CAD build for the part. Positions are in the model's coordinates, mm. Round coordinates to 2 decimals unless told otherwise and drop trailing zeros. Order: outer loops, then holes, each group sorted by start corner. A loop starts at its lowest first (then second) coordinate and runs counter-clockwise, first axis right, second up. Notation, with made-up numbers: M 50.25,72 L 101.25,72 A22 ccw 101.25,94 Z; hole C 30,-28 d5. An arc over 180 degrees is marked long. Answer as a JSON object with one key per item and string values.
```python
from build123d import *

# Parameters (mm, degrees)
SKETCH1_R               = 0.9271
BOSS_EXTRUDE1_DEPTH     = 1.424
BOSS_EXTRUDE2_OUTLINE_R = 0.9271
BOSS_EXTRUDE2_DEPTH     = 0.6096
CUT_EXTRUDE2_START      = -1.424
SKETCH3_R               = 2
CUT_EXTRUDE2_DEPTH      = 2.848


# Read off the part's stored shape, not the designer's step: Boss-Extrude2
with BuildPart() as part:
    # Sketch1 → Boss-Extrude1 (new, symmetric)
    with BuildSketch(Plane(origin=(0, 0, 0), x_dir=(0, 0, -1), z_dir=(1, 0, 0))):
        with BuildLine():
            Line((-3, 2), (3, 2))
            ThreePointArc((3, 2), (5, 0), (3, -2))
            Line((3, -2), (-3, -2))
            ThreePointArc((-3, -2), (-5, 0), (-3, 2))
        make_face()
        with Locations(Location((-3, 0, 0), (0, 0, 180))):
            Circle(SKETCH1_R, mode=Mode.SUBTRACT)
        with Locations(Location((3, 0, 0), (0, 0, 180))):
            Circle(SKETCH1_R, mode=Mode.SUBTRACT)
    extrude(amount=BOSS_EXTRUDE1_DEPTH, both=True)

    # Boss-Extrude2 outline → Boss-Extrude2 (add)
    with BuildSketch(Plane(origin=(1.424, 0, 0), x_dir=(0, 0, -1), z_dir=(1, 0, 0))):
        with BuildLine():
            Line((-3, -2.5019), (3, -2.5019))
            ThreePointArc((3, -2.5019), (5.5019, 0), (3, 2.5019))
            Line((3, 2.5019), (-3, 2.5019))
            ThreePointArc((-3, 2.5019), (-5.5019, 0), (-3, -2.5019))
        make_face()
        with Locations((-3, 0)):
            Circle(BOSS_EXTRUDE2_OUTLINE_R, mode=Mode.SUBTRACT)
        with Locations((3, 0)):
            Circle(BOSS_EXTRUDE2_OUTLINE_R, mode=Mode.SUBTRACT)
    boss_extrude2 = extrude(amount=BOSS_EXTRUDE2_DEPTH)

    # Mirror1: Boss-Extrude2 across plane
    add(boss_extrude2.mirror(Plane(origin=(0, 0, 0), x_dir=(0, 0, 1), z_dir=(1, 0, 0))))

    # Sketch3 → Cut-Extrude2 (cut)
    with BuildSketch(Plane(origin=(0, 0, 0), x_dir=(0, 0, -1), z_dir=(1, 0, 0)).offset(CUT_EXTRUDE2_START)):
        with BuildLine():
            Line((-3, 2.5019), (3, 2.5019))
            ThreePointArc((3, 2.5019), (5.5019, 0), (3, -2.5019))
            Line((3, -2.5019), (-3, -2.5019))
            ThreePointArc((-3, -2.5019), (-5.5019, 0), (-3, 2.5019))
        make_face()
        with Locations(Location((-3, 0, 0), (0, 0, 180))):
            Circle(SKETCH3_R, mode=Mode.SUBTRACT)
        with Locations(Location((3, 0, 0), (0, 0, 180))):
            Circle(SKETCH3_R, mode=Mode.SUBTRACT)
    extrude(amount=CUT_EXTRUDE2_DEPTH, mode=Mode.SUBTRACT)


solid = part.part
```
Item 1: Two-plate mould, pull along Z, no slides. Class faces 1 (the cylindrical face through (-1.7, -0.1, -5.5)), 2 (the flat face through (-1.424, 0, 0)), 3 (the flat face through (-2.034, 0, 0)): released by +Z, released by -Z, zero draft, split by the parting line, or undercut.
Worked answers:
{"face 1": "released by -Z", "face 2": "undercut", "face 3": "zero draft"}
Item 2: Saw through at D-D on y = 1.55. List the corners of the cut face in (x, z), and give its area (3 significant figures).
Worked answers:
{"outline": "M -2.03,-4.96 L -1.42,-4.96 L -1.42,-4.26 L 1.42,-4.26 L 1.42,-4.96 L 2.03,-4.96 L 2.03,4.96 L 1.42,4.96 L 1.42,4.26 L -1.42,4.26 L -1.42,4.96 L -2.03,4.96 Z; hole M -1.42,-1.74 L 1.42,-1.74 L 1.42,1.74 L -1.42,1.74 Z", "area": "26.5 mm2"}
Item 3: Drop flat-ended pins along their axis: pin 1 Ø1.7 at (y, z) = (0, -3) entering from -X; pin 2 Ø2 at (x, z) = (0, -1) entering from -Y; pin 3 Ø2 at (x, z) = (0, 1.5) entering from -Y; pin 4 Ø1 at (x, z) = (-1, -3.5) entering from -Y. Give the stop position or say it passes through.
Worked answers:
{"pin 1": "passes through", "pin 2": "stops at y = -1.73", "pin 3": "stops at y = -1.94", "pin 4": "stops at y = -2.49"}
Item 4: Wall check: line 1 along X through (y, z) = (2.2, -1.5); line 2 along Z through (x, y) = (0.15, 0.05); line 3 along Y through (x, z) = (1.6, 3). Give the ranges that are in metal, low to high. Write a range as [from, to].
Worked answers:
{"line 1": "x = [-2.03, -1.42], [1.42, 2.03]", "line 2": "z = [-5, -3.93], [-2.07, -1], [1, 2.07], [3.93, 5]", "line 3": "y = [-2.5, -0.93], [0.93, 2.5]"}
Item 5: Saw through at C-C on y = 0.6. List the corners of the cut face in (x, z), and give its area (3 significant figures).
Worked answers:
{"outline": "M -2.03,-5.43 L -1.42,-5.43 L -1.42,-4.91 L 1.42,-4.91 L 1.42,-5.43 L 2.03,-5.43 L 2.03,-3.71 L -2.03,-3.71 Z; M -2.03,-2.29 L 2.03,-2.29 L 2.03,2.29 L -2.03,2.29 Z; M -2.03,3.71 L 2.03,3.71 L 2.03,5.43 L 1.42,5.43 L 1.42,4.91 L -1.42,4.91 L -1.42,5.43 L -2.03,5.43 Z; hole M -1.42,-1.09 L 1.42,-1.09 L 1.42,1.09 L -1.42,1.09 Z", "area": "23.5 mm2"}
Item 6: Saw through at A-A on x = 0.2. List the corners of the cut face in (y, z).
Worked answers:
{"outline": "C 0,-3 d4; C 0,3 d4; hole C 0,-3 d1.85; hole C 0,3 d1.85"}
Item 7: Saw through at B-B on z = 0.5. List the corners of the cut face in (x, y), and give its area (3 significant figures).
Worked answers:
{"outline": "M -2.03,-2.5 L -1.42,-2.5 L -1.42,2.5 L -2.03,2.5 Z; M 1.42,-2.5 L 2.03,-2.5 L 2.03,2.5 L 1.42,2.5 Z", "area": "6.10 mm2"}
